```python
from build123d import *

# Parameters (mm, degrees)
BOSS_EXTRUDE1_DEPTH = 60
BOSS_EXTRUDE2_DEPTH = 10
BOSS_EXTRUDE3_DEPTH = 50
SKETCH6_R           = 31
SKETCH6_R_2         = 30
BOSS_EXTRUDE4_DEPTH = 15


with BuildPart() as part:
    # Sketch3 → Boss-Extrude1 (new body)
    with BuildSketch(Plane(origin=(0, 0, 0), x_dir=(1, 0, 0), z_dir=(0, 1, 0))):
        with BuildLine():
            Line((87.760961666, -47.937601186), (113.87798128, -62.699081006))
            Line((113.87798128, -62.699081006), (114.406801927, -63.002726521))
            ThreePointArc((114.406801927, -63.002726521), (125.941479433, -35.014908861), (129.874921777, -5))
            Line((129.874921777, -5), (99.874921777, -5))
            ThreePointArc((99.874921777, -5), (98.598858001, -16.681282954), (95.96133419, -28.132229568))
            ThreePointArc((95.96133419, -28.132229568), (92.393363857, -38.255278265), (87.760961666, -47.937601186))
        make_face()
    extrude(amount=BOSS_EXTRUDE1_DEPTH)

    # Sketch4 → Boss-Extrude2 (add, symmetric)
    with BuildSketch(Plane(origin=(0, 30, 0), x_dir=(1, 0, 0), z_dir=(0, 1, 0))):
        with BuildLine():
            Line((87.760961666, -47.937601186), (65.820721249, -35.95320089))
            ThreePointArc((65.820721249, -35.95320089), (73.538888161, -21.324139043), (76.203852603, -5))
            Line((76.203852603, -5), (99.874921777, -5))
            ThreePointArc((99.874921777, -5), (96.243002799, -27.152981645), (87.760961666, -47.937601186))
        make_face()
    extrude(amount=BOSS_EXTRUDE2_DEPTH, both=True)

    # Sketch5 → Boss-Extrude3 (add, symmetric)
    with BuildSketch(Plane(origin=(0, 30, 0), x_dir=(1, 0, 0), z_dir=(0, 1, 0))):
        with BuildLine():
            Line((129.874921777, -5), (154.874921777, -5))
            Line((154.874921777, -5), (154.874921777, -63.002726521))
            Line((154.874921777, -63.002726521), (154.874921777, -80))
            Line((154.874921777, -80), (114.406801927, -63.002726521))
            ThreePointArc((114.406801927, -63.002726521), (125.941479433, -35.014908861), (129.874921777, -5))
        make_face()
    extrude(amount=BOSS_EXTRUDE3_DEPTH, both=True)

    # Sketch6 → Boss-Extrude4 (add)
    with BuildSketch(Plane(origin=(154.874921777, 0, 0), x_dir=(0, 0, -1), z_dir=(1, 0, 0))):
        with Locations((-42.5, 30)):
            Circle(SKETCH6_R)
        with Locations((-42.5, 30)):
            Circle(SKETCH6_R_2, mode=Mode.SUBTRACT)
    extrude(amount=BOSS_EXTRUDE4_DEPTH)


solid = part.part
```
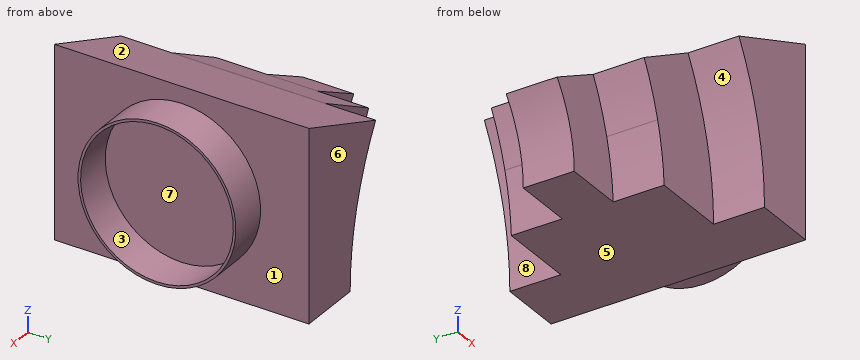
Geometry check sheet. Reference: the model listing, model coordinates, mm. Face numbers are marked on the shaded views. A direction names the side the tool comes from. Round coordinates to 2 decimals unless told otherwise and drop trailing zeros. Order: outer loops, then holes, each group sorted by start corner. A loop starts at its lowest first (then second) coordinate and runs counter-clockwise, first axis right, second up. Notation, with made-up numbers: (-21.75, -27) -> (1.25, -27) arc R23 cw to (1.25, 6) -> close; hole circle Ø10 at (52, 21.25). An arc over 180 degrees is marked (long way). Return JSON: item names as keys, results as strings. Group by question number.
Q1. Gauge pin test, flat ends, axial feed: pin 1 (5 mm diameter, centred on y = 3, z = 43, fed in from +X); pin 2 (8 mm diameter, centred on y = -5.5, z = 47, fed in from -X); pin 3 (2 mm diameter, centred on x = 88, z = 25, fed in from -Y). Record the tip position at first contact, or that the pin passes through.
Q2. Section check D-D, the plane y = 10. Record the boundary of the cut face in (x, z), plus the area to 3 significant figures.
Q3. Material ranges on probe 1 along Y at (x, z) = (158, 42); probe 2 along Y at (x, z) = (73.5, 27.5); probe 3 along Z at (x, y) = (159.5, 24.5), recorded low to high. Write a range as from..to.
Q4. Tool access check on the marked faces 4, 5, 6, 7 and 8. Record the directions out of +Z, -Z, +X, -X, +Y, -Y that give a thin tool (end or side, any length) a straight path to the whole face; none if there is none.
Q5. Release check for a two-part mould opening along Z. For the marked faces 1, 2 and 3 record: released by +Z, released by -Z, zero draft, split by the parting line, or undercut.
Q6. Section check A-A, the plane y = 30. Record the boundary of the cut face in (x, z), plus the area to 3 significant figures.
Q7. Section check B-B, the plane z = 10. Record the boundary of the cut face in (x, y).
Numbers:
{
 "1": {"pin 1": "x = 154.87", "pin 2": "x = 120.41", "pin 3": "y = 20"},
 "2": {"outline": "(87.76, 47.94) arc R100 cw to (99.87, 5) -> (154.87, 5) -> (154.87, 18.81) -> (169.87, 18.81) -> (169.87, 20.14) -> (154.87, 20.14) -> (154.87, 64.86) -> (169.87, 64.86) -> (169.87, 66.19) -> (154.87, 66.19) -> (154.87, 80) -> (114.41, 63) -> (113.88, 62.7) -> close", "area": "3,740 mm^2"},
 "3": {"probe 1": "-1..0, 60..61", "probe 2": "20..40", "probe 3": "11.99..13.01, 71.99..73.01"},
 "4": {"face 4": "-Z, -X, -Y", "face 5": "-Z, +X, -X, +Y, -Y", "face 6": "+Z, -Z, +X, -X, +Y", "face 7": "+X", "face 8": "-Z, -X, +Y"},
 "5": {"face 1": "zero draft", "face 2": "released by +Z", "face 3": "undercut"},
 "6": {"outline": "(65.82, 35.95) arc R51.33 cw to (76.2, 5) -> (154.87, 5) -> (154.87, 11.5) -> (169.87, 11.5) -> (169.87, 12.5) -> (154.87, 12.5) -> (154.87, 72.5) -> (169.87, 72.5) -> (169.87, 73.5) -> (154.87, 73.5) -> (154.87, 80) -> (114.41, 63) -> (113.88, 62.7) -> (87.76, 47.94) -> close", "area": "4,660 mm^2"},
 "7": {"outline": "(75.96, 20) -> (99.5, 20) -> (99.5, 0) -> (129.77, 0) -> (129.77, -20) -> (154.87, -20) -> (154.87, 80) -> (129.77, 80) -> (129.77, 60) -> (99.5, 60) -> (99.5, 40) -> (75.96, 40) -> close"}
}
